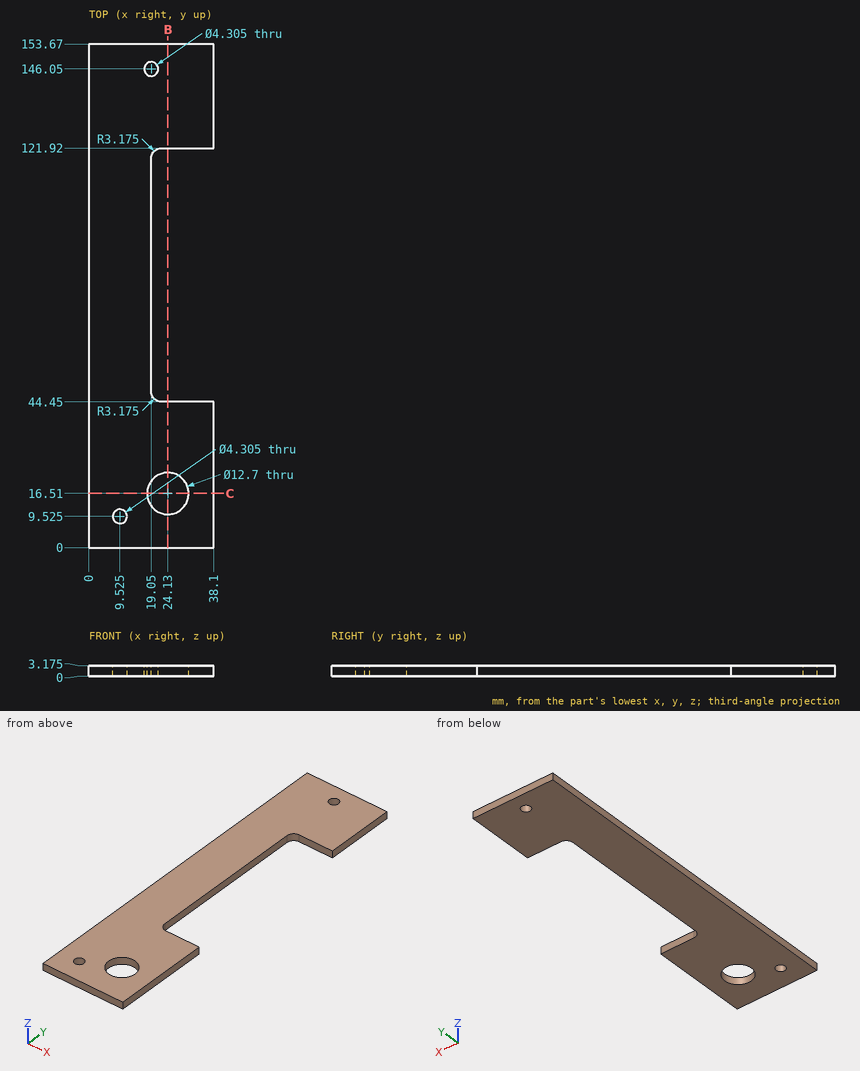
Input: dimensioned drawing with shaded views. Units: mm. Origin: part minimum x, y, z. Give positions to 0.01 mm unless a question says otherwise; leave off trailing zeros. Write each loop counter-clockwise with the first axis right and the second up, starting at its lowest first coordinate (ties: lowest second). Pieces come first, ordered by that corner, then holes.
Q1. Section B-B, the plane x = 24.13. State how many separate pieces and enclosed holes the cut face has, plus the area to 3 significant figures.
Q2. Section C-C, the plane y = 16.51. Output: boundary loops of the cut face in (x, z) (1 decimal).
Q3. Material intervals for probe 1 along Y at (x, z) = (23.5, 2.85); probe 2 along Y at (x, z) = (34, 1.2); probe 3 along Y at (x, z) = (24.13, 1.1), sorted ascending.
Filled in:
1. separate pieces: 3
1. enclosed holes: 0
1. area: 202 mm2
2. outline: (0, 0) - (17.8, 0) - (17.8, 3.2) - (0, 3.2) - close; (30.5, 0) - (38.1, 0) - (38.1, 3.2) - (30.5, 3.2) - close
3. probe 1: y = 0 to 10.19, 22.83 to 44.45, 121.92 to 153.67
3. probe 2: y = 0 to 44.45, 121.92 to 153.67
3. probe 3: y = 0 to 10.16, 22.86 to 44.45, 121.92 to 153.67
